Autodesk Inventor part; units mm, degrees
ref_plane "YZ Plane" through (0, 0, 0) normal (1, 0, 0) x (0, 1, 0)
ref_plane "XZ Plane" through (0, 0, 0) normal (0, 1, 0) x (-1, 0, 0)
ref_plane "XY Plane" through (0, 0, 0) normal (0, 0, 1) x (1, 0, 0)
sketch "Schizzo1" plane through (0, 0, 0) normal (0, 0, 1) x (1, 0, 0)
  point P0 (0, 0)
sketch "Schizzo2" plane through (0, 0, 0) normal (0, 0, 1) x (1, 0, 0)
  line L0 (0, -121) -> (90, -121)
  line L1 (90, -121) -> (90, 0)
  line L2 (0, 0) -> (0, -121)
  line L3 (90, 0) -> (0, 0)
  circle A0 centre (86, -106) radius 2
  circle A1 centre (4, -106) radius 2
  circle A2 centre (4, -6) radius 2
  circle A3 centre (86, -6) radius 2
  line L4 (92, 2) -> (92, -123)
  line L5 (92, -123) -> (-2, -123)
  line L6 (-2, -123) -> (-2, 2)
  line L7 (-2, 2) -> (92, 2)
  dimension "d0" = 2
extrude "Estrusione1" add sketch "Schizzo2" along normal blind 18 contours L4 L5 L6 L7
ref_plane "Piano di lavoro1" through (45, -60.5, 1) normal (0, 0, 1) x (1, 0, 0)
sketch "Schizzo3" plane through (45, -60.5, 1) normal (0, 0, 1) x (1, 0, 0)
  circle A0 centre (41, -45.5) radius 2
  circle A1 centre (-41, -45.5) radius 2
  circle A2 centre (41, 54.5) radius 2
  circle A3 centre (-41, 54.5) radius 2
  line L0 (45, -60.5) -> (45, 60.5)
  line L1 (45, 60.5) -> (-45, 60.5)
  line L2 (-45, -60.5) -> (45, -60.5)
  line L3 (-45, 60.5) -> (-45, -60.5)
  line L4 (-45, -60.5) -> (-45, 60.5)
  line L5 (-39, -41.5) -> (-45, -41.5)
  line L6 (-45, -41.5) -> (-45, -49.5)
  line L7 (-45, -49.5) -> (-39, -49.5)
  line L8 (-37, -47.5) -> (-37, -43.5)
  arc A4 (-37, -43.5) -> (-39, -41.5) centre (-39, -43.5) ccw
  arc A5 (-39, -49.5) -> (-37, -47.5) centre (-39, -47.5) ccw
  line L9 (39, -41.5) -> (45, -41.5)
  line L10 (45, -41.5) -> (45, -49.5)
  line L11 (45, -49.5) -> (39, -49.5)
  line L12 (37, -47.5) -> (37, -43.5)
  arc A6 (37, -47.5) -> (39, -49.5) centre (39, -47.5) ccw
  arc A7 (39, -41.5) -> (37, -43.5) centre (39, -43.5) ccw
  line L13 (37, 60.5) -> (37, 52.5)
  line L14 (39, 50.5) -> (45, 50.5)
  line L15 (45, 50.5) -> (45, 60.5)
  arc A8 (37, 52.5) -> (39, 50.5) centre (39, 52.5) ccw
  line L16 (-45, 60.5) -> (-45, 50.5)
  line L17 (-45, 50.5) -> (-37, 50.5)
  line L18 (-37, 50.5) -> (-37, 60.5)
  point P0 (-45, -41.5)
  point P1 (-45, -49.5)
  point P2 (45, 50.5)
extrude "Estrusione2" add sketch "Schizzo3" along normal blind 2 contours L11 A6 L12 A7 L9 L0 | L3 L5 A4 L8 A5 L7 | L14 A8 L13 L1 L0 | L3 L1 L18 L17
fillet "Raccordo1" radius 2 1 edges at (8, -10, 2)
properties part number "Struttura" material "Plastica ABS"
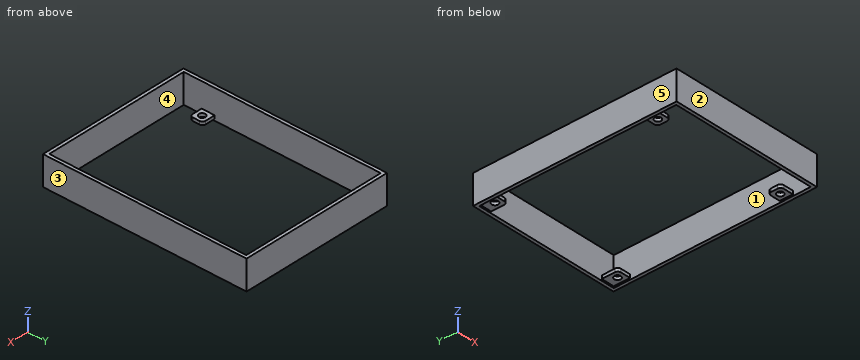
Part model, mm, in its own coordinate system. Face numbers are marked on the shaded views. A direction names the side the tool comes from. Coordinates: 2 decimals unless noted, no trailing zeros. Loops run counter-clockwise (first coordinate to the right, second up) from the corner with the lowest first, then second, coordinate; pieces in that order, holes last. Notation, with made-up numbers: (82, -34.5) - (107, -34.5) arc R23 cw to (107, -12.5) - close; hole circle Ø3 at (12, 72). An arc over 180 degrees is marked (long way). Write item = value, one per line. Start each with the question number.
Item 1: Cut at B-B, the plane y = -6. Give the cut face in (x, z), and give its area (3 significant figures).
Item 2: Mould opens along Y. For the marked faces 1, 2 and 3 say: released by +Y, released by -Y, zero draft, split by the parting line, or undercut.
Item 3: Flat gauge pins, fed straight in: pin 1 Ø6.5 at (x, y) = (86, -104.5) entering from +Z; pin 2 Ø4.5 at (x, y) = (4, -106) entering from -Z; pin 3 Ø3 at (x, y) = (86, -106) entering from +Z. Where does each tip first touch, or does it go through?
Item 4: Cut at C-C, the plane y = -48. Give the cut face in (x, z).
Item 5: Cut at A-A, the plane x = 4. Give the cut face in (y, z).
Item 6: 3-axis set-ups, long thin cutter, end or side, ignore diameter. For the marked faces 4 and 5: which of +Z, -Z, +X, -X, +Y, -Y reach the whole face in a straight line?
Item 7: Wall check: L1, parallel to Y at x = 4, z = 2.05; L2, parallel to Y at x = 9.5, z = 1.5; L3, parallel to X at y = -52.5, z = 16. Give the ranges that are in metal, low to high. Write a range as from..to.
Item 8: Cut at D-D, the plane z = 16. Give the cut face in (x, y).
The answers:
q1.outline = (-2, 0) - (0, 0) - (0, 1) - (2, 1) - (2, 3) - (0, 3) - (0, 18) - (-2, 18) - close; (6, 1) - (8, 1) - (8, 3) - (6, 3) - close; (82, 1) - (84, 1) - (84, 3) - (82, 3) - close; (88, 1) - (90, 1) - (90, 0) - (92, 0) - (92, 18) - (90, 18) - (90, 3) - (88, 3) - close
q1.area = 88.0 mm2
q2.face_1 = undercut
q2.face_2 = released by -Y
q2.face_3 = zero draft
q3.pin_1 = 3
q3.pin_2 = 1
q3.pin_3 = through
q4.outline = (-2, 0) - (0, 0) - (0, 18) - (-2, 18) - close; (90, 0) - (92, 0) - (92, 18) - (90, 18) - close
q5.outline = (-123, 0) - (-121, 0) - (-121, 18) - (-123, 18) - close; (-110, 1) - (-108, 1) - (-108, 3) - (-110, 3) - close; (-104, 1) - (-102, 1) - (-102, 3) - (-104, 3) - close; (-10, 1) - (-8, 1) - (-8, 3) - (-10, 3) - close; (-4, 1) - (0, 1) - (0, 0) - (2, 0) - (2, 18) - (0, 18) - (0, 3) - (-4, 3) - close
q6.face_4 = +Z, -Z
q6.face_5 = +Z, -Z, -X, +Y, -Y
q7.L1 = -123..-121, -110..-108, -104..-102, -10..-8, -4..2
q7.L2 = -123..-121, 0..2
q7.L3 = -2..0, 90..92
q8.outline = (-2, -123) - (92, -123) - (92, 2) - (-2, 2) - close; hole (0, -121) - (90, -121) - (90, 0) - (0, 0) - close
